Check sheet for the modelled part. Datum: model origin and axes. Units: mm. Give positions to 0.01 mm unless a question says otherwise; leave off trailing zeros. Write each loop counter-clockwise with the first axis right and the second up, starting at its lowest first coordinate (ties: lowest second). Pieces come first, ordered by that corner, then holes. Notation, with made-up numbers: (-26, -28.75) -> (-16, -28.75) arc R18 cw to (-16, 1.25) -> close; hole circle Ø6 at (9.25, -21.5). An arc over 180 degrees is marked (long way). Return JSON: item names as keys, results as strings.
from build123d import *

# Parameters (mm, degrees)
F0_R     = 12.7
F0_R_2   = 44.45
F1_DEPTH = 6.35


with BuildPart() as f1:
    # F0 (on Front) → F1 (new body)
    with BuildSketch(Plane.XZ):
        with BuildLine():
            ThreePointArc((-75.117614, -31.731545), (-59.347524, -34.564632), (-46.136719, -43.630874))
            ThreePointArc((-46.136719, -43.630874), (0, -63.5), (46.136719, -43.630874))
            ThreePointArc((46.136719, -43.630874), (59.347524, -34.564632), (75.117614, -31.731545))
            ThreePointArc((75.117614, -31.731545), (107.95, 0), (75.117614, 31.731545))
            ThreePointArc((75.117614, 31.731545), (59.347524, 34.564632), (46.136719, 43.630874))
            ThreePointArc((46.136719, 43.630874), (0, 63.5), (-46.136719, 43.630874))
            ThreePointArc((-46.136719, 43.630874), (-59.347524, 34.564632), (-75.117614, 31.731545))
            ThreePointArc((-75.117614, 31.731545), (-107.95, 0), (-75.117614, -31.731545))
        make_face()
        with Locations((-76.2, 0)):
            Circle(F0_R, mode=Mode.SUBTRACT)
        Circle(F0_R_2, mode=Mode.SUBTRACT)
        with Locations((76.2, 0)):
            Circle(F0_R, mode=Mode.SUBTRACT)
    extrude(amount=-F1_DEPTH)


solid = f1.part
(1) Cross-section at C-C on z = -24. Enter the section's corners in (x, y), then the cut area to 3 significant figures.
Reply:
{"outline": "(-96.99, 0) -> (-37.41, 0) -> (-37.41, 6.35) -> (-96.99, 6.35) -> close; (37.41, 0) -> (96.99, 0) -> (96.99, 6.35) -> (37.41, 6.35) -> close", "area": "757 mm^2"}
(2) Release check for a two-part mould opening along X. For faces 1 (the cylindrical face through (0.723, 3.131, 63.496)), 2 (the cylindrical face through (-64.086, 3.131, 3.815)), 3 (the flat face through (46, 0, 1)) record: pulls with the +X half, pulls with the -X half, needs draft (parallel to the pull), parting line crosses it, or undercut.
Reply:
{"face 1": "parting line crosses it", "face 2": "undercut", "face 3": "needs draft"}
(3) Thickness scan on L1, parallel to Z at x = -76.2, y = 1.5; L2, parallel to X at y = 2.75, z = -11.5; L3, parallel to Z at x = 5, y = 0.5. Record the ranges inside material, lowest first.
Reply:
{"L1": "-31.75 to -12.7, 12.7 to 31.75", "L2": "-105.79 to -81.59, -70.81 to -42.94, 42.94 to 70.81, 81.59 to 105.79", "L3": "-63.3 to -44.17, 44.17 to 63.3"}
(4) Depth check by flat-ended pin: pin 1 Ø2 at (y, z) = (3.5, 38.5) entering from -X; pin 2 Ø2 at (y, z) = (3.5, -0.5) entering from -X. Enter the tip coordinate at first touch or a pass-through.
Reply:
{"pin 1": "x = -53.63", "pin 2": "x = -107.95"}
(5) Cross-section at D-D on y = 1.5. Enter the section's corners in (x, z).
Reply:
{"outline": "(-75.12, -31.73) arc R38.1 cw to (-46.14, -43.63) arc R63.5 ccw to (46.14, -43.63) arc R38.1 cw to (75.12, -31.73) arc R31.75 ccw (long way) to (75.12, 31.73) arc R38.1 cw to (46.14, 43.63) arc R63.5 ccw to (-46.14, 43.63) arc R38.1 cw to (-75.12, 31.73) arc R31.75 ccw (long way) to start; hole circle Ø25.4 at (-76.2, 0); hole circle Ø88.9 at (0, 0); hole circle Ø25.4 at (76.2, 0)"}
(6) Cross-section at B-B on x = 0. Enter the section's corners in (y, z).
Reply:
{"outline": "(0, -63.5) -> (6.35, -63.5) -> (6.35, -44.45) -> (0, -44.45) -> close; (0, 44.45) -> (6.35, 44.45) -> (6.35, 63.5) -> (0, 63.5) -> close"}
(7) Cross-section at A-A on z = 0. Enter the section's corners in (x, y).
Reply:
{"outline": "(-107.95, 0) -> (-88.9, 0) -> (-88.9, 6.35) -> (-107.95, 6.35) -> close; (-63.5, 0) -> (-44.45, 0) -> (-44.45, 6.35) -> (-63.5, 6.35) -> close; (44.45, 0) -> (63.5, 0) -> (63.5, 6.35) -> (44.45, 6.35) -> close; (88.9, 0) -> (107.95, 0) -> (107.95, 6.35) -> (88.9, 6.35) -> close"}
